Geometry check sheet. Reference: drawing and pictorial views, mm from the part's lowest x, y, z. A direction names the side the tool comes from. Round coordinates to 2 decimals unless told otherwise and drop trailing zeros. Write each loop counter-clockwise with the first axis right and the second up, starting at its lowest first coordinate (ties: lowest second). Pieces come first, ordered by that corner, then holes. Notation, with made-up numbers: (73.25, -28.5) -> (113.25, -28.5) arc R31 ccw to (113.25, 1.5) -> close; hole circle Ø5 at (45.5, 58.25). An arc over 180 degrees is marked (long way). Write item = value, one per line.
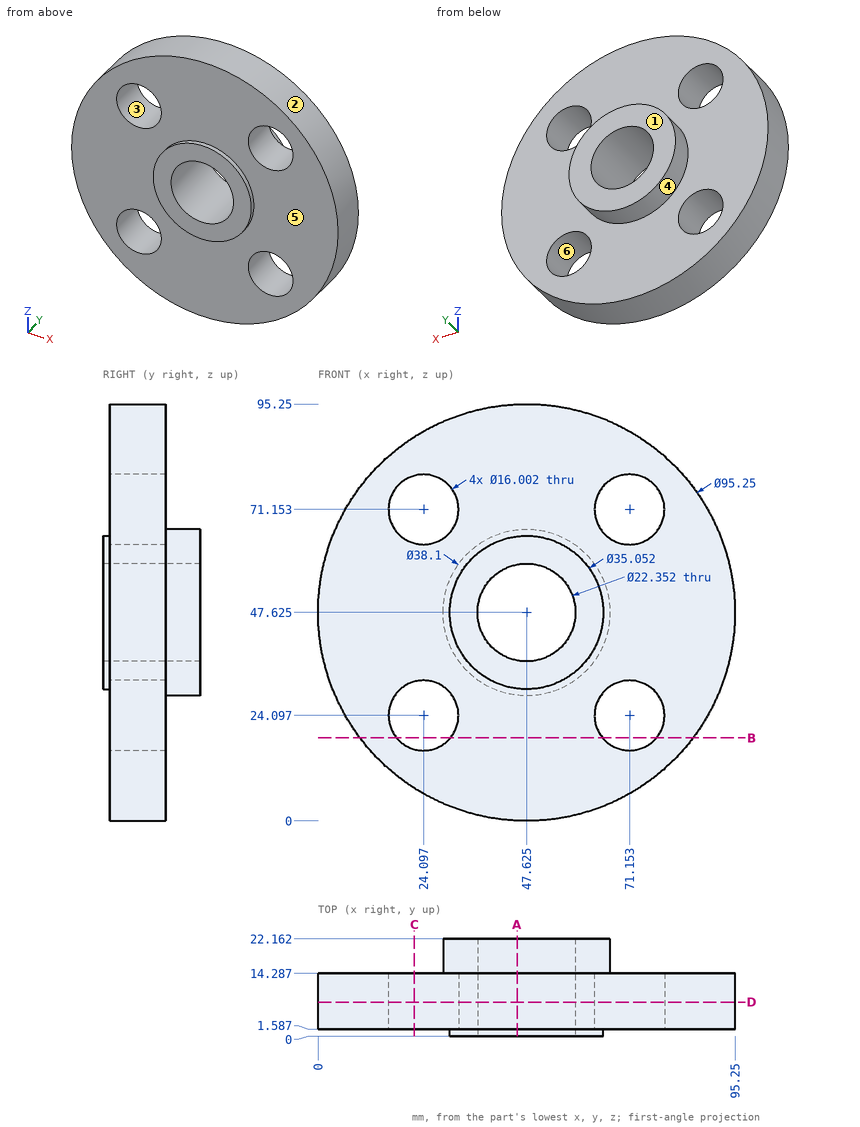
(1) Sectioned sample at C-C on x = 22. Enter the section's corners in (y, z) (1 decimal).
Worked answers:
outline = (1.6, 7.5) -> (14.3, 7.5) -> (14.3, 16.4) -> (1.6, 16.4) -> close; (1.6, 31.8) -> (14.3, 31.8) -> (14.3, 63.4) -> (1.6, 63.4) -> close; (1.6, 78.9) -> (14.3, 78.9) -> (14.3, 87.8) -> (1.6, 87.8) -> close
(2) Material ranges on L1, parallel to X at y = 8.25, z = 19 (1 decimal); L2, parallel to Y at x = 77.5, z = 38; L3, parallel to X at y = 17.5, z = 48 (1 decimal), recorded low to high. Write a range as [from, to].
Worked answers:
L1 = [9.6, 17.9], [30.3, 65], [77.3, 85.7]
L2 = [1.59, 14.29]
L3 = [28.6, 36.5], [58.8, 66.7]
(3) Go/stop test with flat-tipped pins: P1, Ø2, axis at x = 39, z = 18, coming from the -Y side; P2, Ø10, axis at x = 77, z = 52, coming from the +Y side; P3, Ø1.5, axis at x = 37, y = 19, coming from the +Z side (1 decimal); P4, Ø18, axis at x = 47.625, z = 47.625, coming from the +Y side. Record where each tip stops, or that it passes through.
Worked answers:
P1 = 1.59
P2 = 14.29
P3 = 63.9
P4 = through
(4) Release check for a two-part mould opening along X. For the marked faces 1, 2 and 3 record: pulls with the +X half, pulls with the -X half, needs draft (parallel to the pull), parting line crosses it, or undercut.
Worked answers:
face_1 = needs draft
face_2 = parting line crosses it
face_3 = undercut
(5) Sectioned sample at D-D on y = 7.75. Count the separate pieces of the cut face and the enclosed holes in it, then the cut area to 3 significant figures.
Worked answers:
separate_pieces = 1
enclosed_holes = 5
area = 5,930 mm²
(6) Sectioned sample at A-A on x = 45.5. Enter the section's corners in (y, z), then the cut area to 3 significant figures.
Worked answers:
outline = (0, 30.23) -> (1.59, 30.23) -> (1.59, 0.05) -> (14.29, 0.05) -> (14.29, 28.69) -> (22.16, 28.69) -> (22.16, 36.65) -> (0, 36.65) -> close; (0, 58.6) -> (22.16, 58.6) -> (22.16, 66.56) -> (14.29, 66.56) -> (14.29, 95.2) -> (1.59, 95.2) -> (1.59, 65.02) -> (0, 65.02) -> close
area = 1,080 mm²
(7) Access from +Z, -Z, +X, -X, +Y, -Y to the whole of each face (thin tool, end or side, straight path). Record for the marked faces 4, 5 and 6.
Worked answers:
face_4 = +Y
face_5 = -Y
face_6 = +Y, -Y
(8) Sectioned sample at B-B on z = 19. Enter the section's corners in (x, y) (1 decimal).
Worked answers:
outline = (9.6, 1.6) -> (17.9, 1.6) -> (17.9, 14.3) -> (9.6, 14.3) -> close; (30.3, 1.6) -> (65, 1.6) -> (65, 14.3) -> (30.3, 14.3) -> close; (77.3, 1.6) -> (85.7, 1.6) -> (85.7, 14.3) -> (77.3, 14.3) -> close
